For this review, take the finished solid that the model builds, in its own axes (mm). Face numbers are marked on the shaded views. A direction names the side the tool comes from. Coordinates: 2 decimals unless noted, no trailing zeros. Write each loop counter-clockwise with the first axis right and the second up, starting at its lowest first coordinate (ties: lowest second). Pieces come first, ordered by that corner, then holes. Notation, with made-up numbers: (52.5, 27) - (111.5, 27) arc R11 cw to (111.5, 40) - close; hole circle Ø8 at (86.25, 24). An arc over 180 degrees is marked (long way). Use one line per item in the form item = value. Start each with the question number.
1) Mouldability with a two-part tool opening along X and no side actions: class the marked faces 3, 4, 5 and 6 as pulls with the +X half, pulls with the -X half, needs draft (parallel to the pull), parting line crosses it, or undercut.
2) We need section A-A (x = 0). Give the boundary of the cut face in (y, z), plus the area to 3 significant figures.
3) We need section D-D (x = 1.75). Give the boundary of the cut face in (y, z), plus the area to 3 significant figures.
4) For L1, parallel to Y at x = 1.5, z = -2.25; L2, parallel to Z at x = -0.75, y = 7; L3, parallel to X at y = 7.25, z = 0, list the stretches that pass through material, from the lowest coordinate up. Write a range as from..to.
5) Insertion check: P1, Ø1.5, axis at x = -2.5, z = -1.5, coming from the +Y side. The pin has a flat end and moves straight along its axis. Give the tip position at first contact, or say it passes through.
6) Tool access review of the marked faces 1 and 2: name each direction out of +Z, -Z, +X, -X, +Y, -Y from which nothing blocks a thin tool from reaching the whole face with its end or side.
7) We need section C-C (z = -0.25). Give the boundary of the cut face in (x, y), plus the area to 3 significant figures.
```python
from build123d import *

# Parameters (mm, degrees)
BOSS_EXTRUDE1_DEPTH = 3.81
SKETCH2_R           = 2.032
BOSS_EXTRUDE2_DEPTH = 5.08
CUT_EXTRUDE1_DEPTH  = 9.89


with BuildPart() as part:
    # Sketch1 → Boss-Extrude1 (new body)
    with BuildSketch(Plane(origin=(0, 0, 0), x_dir=(1, 0, 0), z_dir=(0, 1, 0))):
        Polygon((6.35, 0), (3.175, 5.499261314), (-3.175, 5.499261314), (-6.35, 0), (-3.175, -5.499261314), (3.175, -5.499261314), align=None)
    extrude(amount=BOSS_EXTRUDE1_DEPTH)

    # Sketch2 → Boss-Extrude2 (add)
    with BuildSketch(Plane(origin=(0, 3.81, 0), x_dir=(1, 0, 0), z_dir=(0, 1, 0))):
        Circle(SKETCH2_R)
    extrude(amount=BOSS_EXTRUDE2_DEPTH)

    # Sketch3 → Cut-Extrude1 (cut, through all)
    with BuildSketch(Plane.XZ):
        with BuildLine():
            Line((-1.062558234, -0.5715), (1.062558234, -0.5715))
            ThreePointArc((1.062558234, -0.5715), (0, 1.2065), (-1.062558234, -0.5715))
        make_face()
    extrude(amount=-CUT_EXTRUDE1_DEPTH, mode=Mode.SUBTRACT)


solid = part.part
```
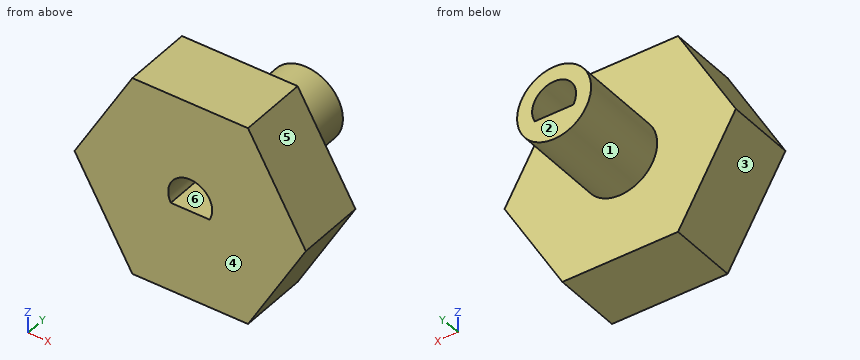
Determined:
q1.face_3 = pulls with the -X half
q1.face_4 = needs draft
q1.face_5 = pulls with the +X half
q1.face_6 = undercut
q2.outline = (0, -5.5) - (3.81, -5.5) - (3.81, -2.03) - (8.89, -2.03) - (8.89, -0.57) - (0, -0.57) - close; (0, 1.21) - (8.89, 1.21) - (8.89, 2.03) - (3.81, 2.03) - (3.81, 5.5) - (0, 5.5) - close
q2.area = 46.7 mm²
q3.outline = (0, -5.5) - (3.81, -5.5) - (3.81, -1.03) - (8.89, -1.03) - (8.89, 1.03) - (3.81, 1.03) - (3.81, 5.5) - (0, 5.5) - close
q3.area = 52.4 mm²
q4.L1 = 0..3.81
q4.L2 = -1.89..-0.57, 0.95..1.89
q4.L3 = -2.03..-1.21, 1.21..2.03
q5.P1 = 3.81
q6.face_1 = +Y
q6.face_2 = +Z, -Z, +X, -X, +Y
q7.outline = (-6.21, 0) - (-1.18, 0) - (-1.18, 8.89) - (-2.02, 8.89) - (-2.02, 3.81) - (-6.21, 3.81) - close; (1.18, 0) - (6.21, 0) - (6.21, 3.81) - (2.02, 3.81) - (2.02, 8.89) - (1.18, 8.89) - close
q7.area = 46.8 mm²
